from build123d import *


with BuildPart() as part:
    # Sketch1 → Revolve1 (revolve)
    with BuildSketch(Plane.XY, mode=Mode.PRIVATE) as revolve1_sk:
        with BuildLine():
            Line((-6, 10), (6, 10))
            ThreePointArc((6, 10), (6.707106781, 10.292893219), (7, 11))
            Line((7, 11), (7, 14.15))
            Line((7, 14.15), (5.04, 14.15))
            Line((5.04, 14.15), (5.04, 14.4))
            Line((5.04, 14.4), (2.856571371, 14.4))
            ThreePointArc((2.856571371, 14.4), (0, 13.2), (-2.856571371, 14.4))
            Line((-2.856571371, 14.4), (-5.04, 14.4))
            Line((-5.04, 14.4), (-5.04, 14.15))
            Line((-5.04, 14.15), (-7, 14.15))
            Line((-7, 14.15), (-7, 11))
            ThreePointArc((-7, 11), (-6.707106781, 10.292893219), (-6, 10))
        make_face()
    revolve(revolve1_sk.sketch.rotate(Axis((0, 0, 0), (-1, 0, 0)), 90), axis=Axis((0, 0, 0), (-1, 0, 0)))


solid = part.part
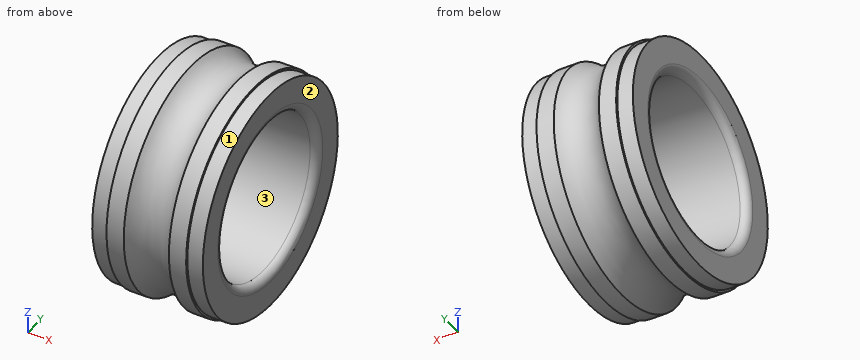
Source: CAD feature listing. Evaluate the final solid. Frame: model axes, mm. Face numbers are marked on the shaded views. Round coordinates to 2 decimals unless told otherwise and drop trailing zeros. Write each loop counter-clockwise with the first axis right and the second up, starting at its lowest first coordinate (ties: lowest second). Pieces come first, ordered by that corner, then holes. Notation, with made-up numbers: M -33.75,-20.5 L -19.75,-20.5 A5 cw -19.75,-13.5 Z; hole C 80,18.5 d8. An arc over 180 degrees is marked long. One line per item, written item: value. Start each with the question number.
Item 1: Mould query, pull axis Z, two halves, no side actions, for the marked faces 1, 2 and 3. Classes: pulls with the +Z half, pulls with the -Z half, needs draft (parallel to the pull), parting line crosses it, or undercut.
Item 2: Section query C-C (x = 4). Return the cut outline in (y, z), plus the area to 3 significant figures.
Item 3: Section query D-D (x = -5.5). Return the cut outline in (y, z), plus the area to 3 significant figures.
Item 4: Section query A-A (z = 0). Return the cut outline in (x, y), plus the area to 3 significant figures.
Item 5: Pin query (flat end, axial travel): pin 1 (3 mm diameter, centred on y = -8, z = 4.5, fed in from +X); pin 2 (1 mm diameter, centred on x = 2, z = -9.5, fed in from +Y); pin 3 (5 mm diameter, centred on x = -5, z = 10, fed in from +Y). Return the tip coordinate at first contact, or that it passes through.
Item 6: Ray query, L1, parallel to Y at x = -3, z = 0; L2, parallel to Y at x = 2, z = 0; L3, parallel to Z at x = -0.5, y = -7.75. Return the intervals inside material, ascending. Write a range as from..to.
Result set:
1. face 1: parting line crosses it
1. face 2: needs draft
1. face 3: undercut
2. outline: C 0,0 d28.8; hole C 0,0 d20
2. area: 337 mm²
3. outline: C 0,0 d28.3; hole C 0,0 d20
3. area: 315 mm²
4. outline: M -7,-14.15 L -5.04,-14.15 L -5.04,-14.4 L -2.86,-14.4 A4 cw 2.86,-14.4 L 5.04,-14.4 L 5.04,-14.15 L 7,-14.15 L 7,-11 A1 ccw 6,-10 L -6,-10 A1 ccw -7,-11 Z; M -7,11 A1 ccw -6,10 L 6,10 A1 ccw 7,11 L 7,14.15 L 5.04,14.15 L 5.04,14.4 L 2.86,14.4 A4 cw -2.86,14.4 L -5.04,14.4 L -5.04,14.15 L -7,14.15 Z
4. area: 111 mm²
5. pin 1: stops at x = 6.95
5. pin 2: stops at y = 10.55
5. pin 3: stops at y = 12.29
6. L1: y = -14.4..-10, 10..14.4
6. L2: y = -13.74..-10, 10..13.74
6. L3: z = -10.72..-6.32, 6.32..10.72
